```python
from build123d import *

# Parameters (mm, degrees)
SKETCH1_W           = 100
SKETCH1_H           = 26
BOSS_EXTRUDE1_DEPTH = 2
BOSS_EXTRUDE2_DEPTH = 100
SKETCH3_W           = 25
SKETCH3_H           = 28
BOSS_EXTRUDE3_DEPTH = 4
SKETCH4_R           = 2.1
CUT_EXTRUDE1_DEPTH  = 106.39449701
MOVE_FACE1_BY       = 2
MOVE_FACE1_2_BY     = 2
SKETCH5_R           = 3.6
CUT_EXTRUDE2_DEPTH  = 4.2
MOVE_FACE2_BY       = 4
MOVE_FACE3_BY       = 3.8


with BuildPart() as part:
    # Sketch1 → Boss-Extrude1 (new body)
    with BuildSketch(Plane(origin=(0, 0, 0), x_dir=(0, 0, -1), z_dir=(1, 0, 0))):
        with Locations((50, 13)):
            Rectangle(SKETCH1_W, SKETCH1_H)
    extrude(amount=BOSS_EXTRUDE1_DEPTH)

    # Sketch2 → Boss-Extrude2 (add)
    with BuildSketch(Plane.XY):
        Polygon((2, 26), (2, 28), (-12, 28), (-12, 24), (-10, 24), (-10, 26), align=None)
    extrude(amount=-BOSS_EXTRUDE2_DEPTH)

    # Sketch3 → Boss-Extrude3 (add)
    with BuildSketch(Plane(origin=(2, 0, 0), x_dir=(0, 0, -1), z_dir=(1, 0, 0))):
        with Locations((50, 14)):
            Rectangle(SKETCH3_W, SKETCH3_H)
    extrude(amount=BOSS_EXTRUDE3_DEPTH)

    # Sketch4 → Cut-Extrude1 (cut, through all)
    with BuildSketch(Plane(origin=(6, 0, 0), x_dir=(0, 0, -1), z_dir=(1, 0, 0))):
        with Locations((41.5, 21)):
            Circle(SKETCH4_R)
        with Locations((58.5, 21)):
            Circle(SKETCH4_R)
        with Locations((58.5, 4)):
            Circle(SKETCH4_R)
        with Locations((41.5, 4)):
            Circle(SKETCH4_R)
    extrude(amount=-CUT_EXTRUDE1_DEPTH, mode=Mode.SUBTRACT)

    # Move Face1: a face moved outward by 2.0
    extrude(part.faces().sort_by_distance((4, 14, -37.5))[0], amount=MOVE_FACE1_BY, dir=(0, 0, 1))

    # Move Face1 2: a face moved outward by 2.0
    extrude(part.faces().sort_by_distance((4, 14, -62.5))[0], amount=MOVE_FACE1_2_BY, dir=(0, 0, -1))

    # Sketch5 → Cut-Extrude2 (cut)
    with BuildSketch(Plane.ZY):
        with Locations((-58.5, 21)):
            Circle(SKETCH5_R)
        with Locations((-41.5, 21)):
            Circle(SKETCH5_R)
        with Locations((-41.5, 4)):
            Circle(SKETCH5_R)
        with Locations((-58.5, 4)):
            Circle(SKETCH5_R)
    extrude(amount=-CUT_EXTRUDE2_DEPTH, mode=Mode.SUBTRACT)

    # Move Face2: a face moved outward by 4.0
    extrude(part.faces().sort_by_distance((6, 14.109871115, -50))[0], amount=MOVE_FACE2_BY, dir=(1, 0, 0))

    # Move Face3: a face moved inward by 3.8
    extrude(part.faces().sort_by_distance((10, 14.109871115, -50))[0], amount=MOVE_FACE3_BY, dir=(-1, 0, 0), mode=Mode.SUBTRACT)


solid = part.part
```
Here's how the part is built. I have some questions about the finished solid (model axes, mm). A direction names the side the tool comes from. Coordinates: 2 decimals unless noted, no trailing zeros. Order: outer loops, then holes, each group sorted by start corner. A loop starts at its lowest first (then second) coordinate and runs counter-clockwise, first axis right, second up.
1) Imagine slicing it at A-A on y = 4. List the corners of the cut face in (x, z) for me.
2) I need wall thicknesses on line 1 (Y direction, x = 6.1, z = -41.5); line 2 (Y direction, x = 3.3, z = -41.5); line 3 (Z direction, x = 1.5, y = 3.25). Which ranges of each line are inside material? Lowest first, please.
3) Imagine slicing it at B-B on z = -41.5. List the corners of the cut face in (x, y) for me, and give its area (3 significant figures).
4) Which directions (+Z, -Z, +X, -X, +Y, -Y) give clear straight access to the entire face, cutting with the end or side of a thin tool? Please do faces 4 (the face through (-10, 25, -49)), 5 (the face through (2.071, 19.621, -55.175)), 6 (the face through (2.071, 5.081, -55.066)).
5) We'd pull the mould along X, two halves only. Please class faces 1 (the face through (2, 14, -18)), 2 (the face through (2.071, 17.486, -42.28)), 3 (the face through (4.2, 2, -57)): +X half, -X half, draft (parallel to the pull), parting line (faces both ways), or undercut.
6) Imagine slicing it at C-C on z = -78.5. List the corners of the cut face in (x, y) for me, and give its area (3 significant figures).
7) Imagine slicing it at D-D on y = 9.5. List the corners of the cut face in (x, z) for me, and give its area (3 significant figures).
8) Will these pins go through, and if not, where does the flat tip stop? pin 1 (1 mm diameter, centred on x = -5, z = -31.5, fed in from -Y); pin 2 (0.6 mm diameter, centred on x = -11, z = -64, fed in from -Y); pin 3 (6.5 mm diameter, centred on y = 21, z = -41.5, fed in from +X); pin 4 (9.5 mm diameter, centred on y = 4, z = -41.5, fed in from -X).
Response values:
1. outline: (0, -100) - (2, -100) - (2, -64.5) - (6.2, -64.5) - (6.2, -60.6) - (4.2, -60.6) - (4.2, -62.1) - (0, -62.1) - close; (0, -54.9) - (4.2, -54.9) - (4.2, -56.4) - (6.2, -56.4) - (6.2, -43.6) - (4.2, -43.6) - (4.2, -45.1) - (0, -45.1) - close; (0, -37.9) - (4.2, -37.9) - (4.2, -39.4) - (6.2, -39.4) - (6.2, -35.5) - (2, -35.5) - (2, 0) - (0, 0) - close
2. line 1: y = 0 to 1.9, 6.1 to 18.9, 23.1 to 28
2. line 2: y = 0 to 0.4, 7.6 to 17.4, 24.6 to 28
2. line 3: z = -100 to -62.02, -54.98 to -45.02, -37.98 to 0
3. outline: (-12, 24) - (-10, 24) - (-10, 26) - (0, 26) - (0, 24.6) - (4.2, 24.6) - (4.2, 23.1) - (6.2, 23.1) - (6.2, 28) - (-12, 28) - close; (0, 0) - (6.2, 0) - (6.2, 1.9) - (4.2, 1.9) - (4.2, 0.4) - (0, 0.4) - close; (0, 7.6) - (4.2, 7.6) - (4.2, 6.1) - (6.2, 6.1) - (6.2, 18.9) - (4.2, 18.9) - (4.2, 17.4) - (0, 17.4) - close
3. area: 124 mm2
4. face 4: +Z, -Z, -Y
4. face 5: none
4. face 6: -X
5. face 1: +X half
5. face 2: undercut
5. face 3: -X half
6. outline: (-12, 24) - (-10, 24) - (-10, 26) - (0, 26) - (0, 0) - (2, 0) - (2, 28) - (-12, 28) - close
6. area: 84.0 mm2
7. outline: (0, -100) - (2, -100) - (2, -64.5) - (6.2, -64.5) - (6.2, -35.5) - (2, -35.5) - (2, 0) - (0, 0) - close
7. area: 322 mm2
8. pin 1: stops at y = 26
8. pin 2: stops at y = 24
8. pin 3: stops at x = 6.2
8. pin 4: stops at x = 0
